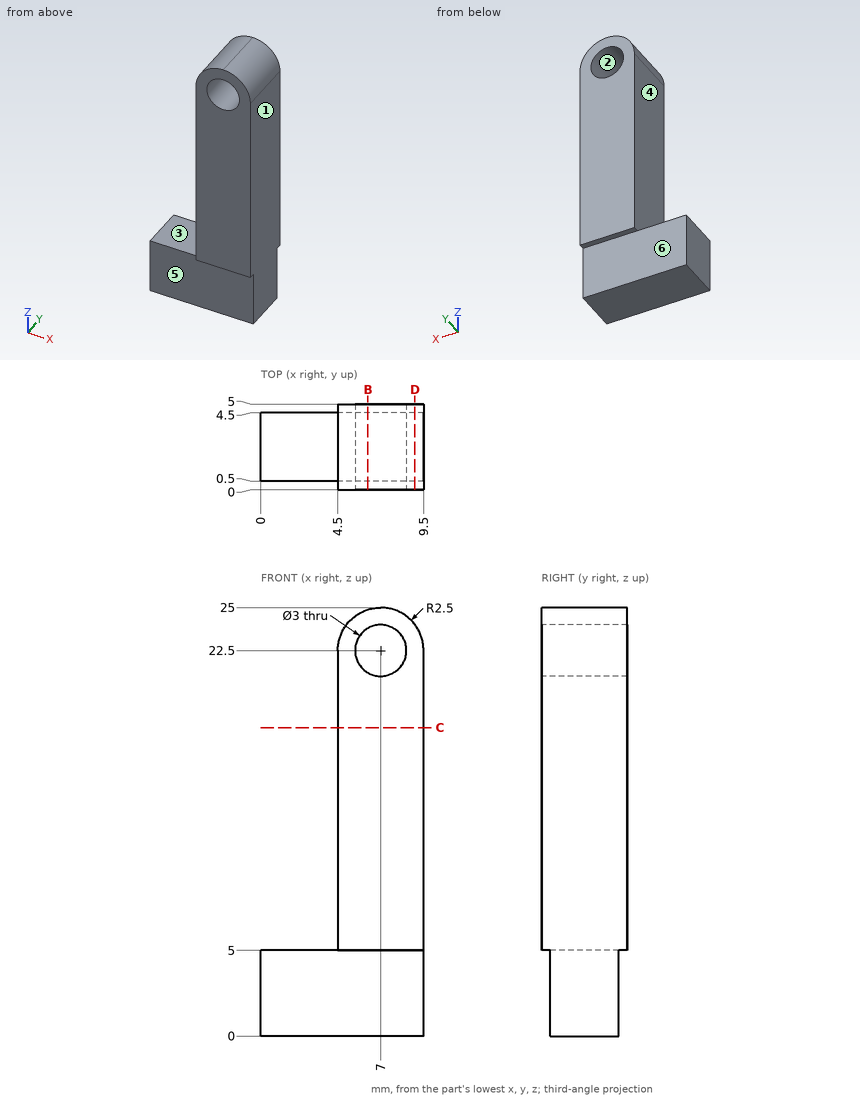
Print and shaded views of the part. All mm, measured from the part's lowest x, y and z. A direction names the side the tool comes from. Give positions to 0.01 mm unless a question says otherwise; leave off trailing zeros. Loops run counter-clockwise (first coordinate to the right, second up) from the corner with the lowest first, then second, coordinate; pieces in that order, holes last. Notation, with made-up numbers: (-30, 27.5) - (-8, 27.5) arc R31 ccw to (-8, 63.5) - close; hole circle Ø7 at (19.5, -4.75). An arc over 180 degrees is marked (long way). One line per item, written item: value. Start each with the question number.
1. Slice it at C-C (z = 18). List the corners of the cut face in (x, y), plus the area to 3 significant figures.
2. Slice it at D-D (x = 9). List the corners of the cut face in (y, z), plus the area to 3 significant figures.
3. Pull direction Z, two halves, no side cores. Call the marked faces 1, 2 and 3: pulls with the +Z half, pulls with the -Z half, needs draft (parallel to the pull), parting line crosses it, or undercut.
4. Slice it at B-B (x = 6.25). List the corners of the cut face in (y, z), plus the area to 3 significant figures.
5. Which spindle directions (+Z, -Z, +X, -X, +Y, -Y) get a long thin tool onto all of the face, cutting with end or side? Do the marked faces 4, 5 and 6. Say none if no direction does.
6. Probe L1, parallel to Z at x = 7, y = 3.5; L2, parallel to X at y = 2.95, z = 22.5; L3, parallel to Y at x = 9, z = 3.25. List the from-to ranges inside material, lowest first. Write a range as from..to.
7. Pin check, flat tips, straight feed: pin 1 (1.5 mm diameter, centred on x = 2, z = 3.5, fed in from -Y); pin 2 (1.2 mm diameter, centred on x = 2.5, y = 3.5, fed in from +Z). Stop position of each tip, or through.
Solution:
1. outline: (4.5, 0) - (9.5, 0) - (9.5, 5) - (4.5, 5) - close
1. area: 25.0 mm^2
2. outline: (0, 5) - (0.5, 5) - (0.5, 0) - (4.5, 0) - (4.5, 5) - (5, 5) - (5, 24) - (0, 24) - close
2. area: 115 mm^2
3. face 1: needs draft
3. face 2: undercut
3. face 3: pulls with the +Z half
4. outline: (0, 5) - (0.5, 5) - (0.5, 0) - (4.5, 0) - (4.5, 5) - (5, 5) - (5, 21.2) - (0, 21.2) - close; (0, 23.8) - (5, 23.8) - (5, 24.88) - (0, 24.88) - close
4. area: 106 mm^2
5. face 4: +Z, -X, +Y, -Y
5. face 5: -Z, +X, -X, -Y
5. face 6: -Z, +X, -X, +Y
6. L1: z = 0..21, 24..25
6. L2: x = 4.5..5.5, 8.5..9.5
6. L3: y = 0.5..4.5
7. pin 1: stops at y = 0.5
7. pin 2: stops at z = 5
